The model under review builds one solid part; all positions refer to its coordinate system, in mm. A direction names the side the tool comes from. Give positions to 0.01 mm unless a question says otherwise; leave off trailing zeros. Loops run counter-clockwise (first coordinate to the right, second up) from the corner with the lowest first, then second, coordinate; pieces in that order, holes last. Notation, with made-up numbers: (68.5, -30) -> (94.5, -30) arc R13 ccw to (94.5, -11) -> close; hole circle Ø9 at (62.5, -22.5). An arc over 180 degrees is marked (long way). Write each question's results on one line, items separated by ' | '. Start each with the question number.
Q1. We need section A-A (y = 37). Write out the cut boundary in (x, z).
Q2. Wall thickness on L1, parallel to Z at x = -3, y = 21; L2, parallel to Z at x = 6.5, y = 237.5: over which ranges is each line inside the solid? List them lowest first. Write a range as [from, to].
Q3. Insertion check: pin 1 Ø4 at (x, y) = (0, 15) entering from +Z; pin 2 Ø1.8 at (x, y) = (0, 30) entering from -Z. Each pin has a flat end and moves straight along its axis. Give the tip position at first contact, or say it passes through.
Q4. Mouldability with a two-part tool opening along X and no side actions: class faces 3 (the face through (7.5, 118, 0)), 4 (the face through (-7, 0, 0)), 5 (the face through (5.5, 122, 0)), 6 (the face through (-7.5, 118, 0)) as released by +X, released by -X, zero draft, split by the parting line, or undercut.
Q5. Machinability: for faces 1 (the face through (-5.5, 122, 0)), 2 (the face through (6, 35, 0)), which of the approach directions +Z, -Z, +X, -X, +Y, -Y give a long, thin tool a straight path to every point of the face, cutting with its end or side? Answer none if there is none.
Q6. We need section B-B (y = 119.5). Write out the cut boundary in (x, z).
from build123d import *

# Parameters (mm, degrees)
SKETCH_1_W          = 15
SKETCH_1_H          = 15
EXTRUDE_1_DEPTH     = 240
SKETCH_2_W          = 11
SKETCH_2_H          = 11
CUT_EXTRUDE_1_DEPTH = 240
SKETCH_3_R          = 2.5
CUT_EXTRUDE_2_DEPTH = 15
SKETCH_4_R          = 1.5
CUT_EXTRUDE_3_DEPTH = 15
SKETCH_5_R          = 1.5
SKETCH_5_R_2        = 2
CUT_EXTRUDE_4_DEPTH = 15


with BuildPart() as part:
    # 草图1 → 凸台-拉伸1 (new body)
    with BuildSketch(Plane(origin=(0, 0, 0), x_dir=(1, 0, 0), z_dir=(0, 1, 0))):
        Rectangle(SKETCH_1_W, SKETCH_1_H)
    extrude(amount=EXTRUDE_1_DEPTH)

    # 草图2 → 切除-拉伸1 (cut)
    with BuildSketch(Plane(origin=(0, 240, 0), x_dir=(1, 0, 0), z_dir=(0, 1, 0))):
        Rectangle(SKETCH_2_W, SKETCH_2_H)
    extrude(amount=-CUT_EXTRUDE_1_DEPTH, mode=Mode.SUBTRACT)

    # 草图3 → 切除-拉伸2 (cut)
    with BuildSketch(Plane.XY.offset(7.5)):
        with Locations((0, 140)):
            Circle(SKETCH_3_R)
        with Locations((0, 100)):
            Circle(SKETCH_3_R)
    extrude(amount=-CUT_EXTRUDE_2_DEPTH, mode=Mode.SUBTRACT)

    # 草图4 → 切除-拉伸3 (cut)
    with BuildSketch(Plane.XY.offset(7.5)):
        with Locations((0, 45)):
            Circle(SKETCH_4_R)
        with Locations((0, 30)):
            Circle(SKETCH_4_R)
        with Locations((0, 15)):
            Circle(SKETCH_4_R)
    extrude(amount=-CUT_EXTRUDE_3_DEPTH, mode=Mode.SUBTRACT)

    # 草图5 → 切除-拉伸4 (cut)
    with BuildSketch(Plane.ZY.offset(7.5)):
        with Locations((0, 10)):
            Circle(SKETCH_5_R)
        with Locations((0, 37)):
            Circle(SKETCH_5_R_2)
        with Locations((0, 50)):
            Circle(SKETCH_5_R)
        with Locations((0, 237.5)):
            Circle(SKETCH_5_R)
        with Locations((0, 217.5)):
            Circle(SKETCH_5_R)
        with Locations((0, 197.5)):
            Circle(SKETCH_5_R)
    extrude(amount=-CUT_EXTRUDE_4_DEPTH, mode=Mode.SUBTRACT)


solid = part.part
Output:
1) outline: (-7.5, -7.5) -> (7.5, -7.5) -> (7.5, -2) -> (5.5, -2) -> (5.5, -5.5) -> (-5.5, -5.5) -> (-5.5, -2) -> (-7.5, -2) -> close; (-7.5, 2) -> (-5.5, 2) -> (-5.5, 5.5) -> (5.5, 5.5) -> (5.5, 2) -> (7.5, 2) -> (7.5, 7.5) -> (-7.5, 7.5) -> close
2) L1: [-7.5, -5.5], [5.5, 7.5] | L2: [-7.5, -1.5], [1.5, 7.5]
3) pin 1: z = 7.5 | pin 2: through
4) face 3: released by +X | face 4: zero draft | face 5: undercut | face 6: released by -X
5) face 1: +Y, -Y | face 2: +X, -X
6) outline: (-7.5, -7.5) -> (7.5, -7.5) -> (7.5, 7.5) -> (-7.5, 7.5) -> close; hole (-5.5, -5.5) -> (5.5, -5.5) -> (5.5, 5.5) -> (-5.5, 5.5) -> close
